Geometry check sheet. Reference: drawing and pictorial views, mm from the part's lowest x, y, z. A direction names the side the tool comes from. Round coordinates to 2 decimals unless told otherwise and drop trailing zeros. Write each loop counter-clockwise with the first axis right and the second up, starting at its lowest first coordinate (ties: lowest second). Pieces come first, ordered by that corner, then holes.
Item 1: Material ranges on line 1 along Y through (x, z) = (2.75, 3.25); line 2 along Z through (x, y) = (5.75, 1) (1 decimal); line 3 along X through (y, z) = (1.5, 6), recorded low to high.
Item 2: Section check D-D, the plane z = 4.25. Record the cut outline in (x, y).
Item 3: Section check C-C, the plane z = 6. Record the cut outline in (x, y).
Item 4: Release check for a two-part mould opening along Z. For the marked faces 3, 4, 5 and 6 record: pulls with the +Z half, pulls with the -Z half, needs draft (parallel to the pull), parting line crosses it, or undercut.
Item 5: Set-up check for the marked faces 1 and 2: record each of +Z, -Z, +X, -X, +Y, -Y from which the full face is reachable in a straight line by a thin tool's end or side.
Item 6: Depth check by flat-ended pin: pin 1 (3 mm diameter, centred on x = 6, y = 6.5, fed in from -Z). Enter the tip coordinate at first touch or a pass-through.
Item 7: Section check A-A, the plane x = 6.35. Record the cut outline in (y, z) (1 decimal).
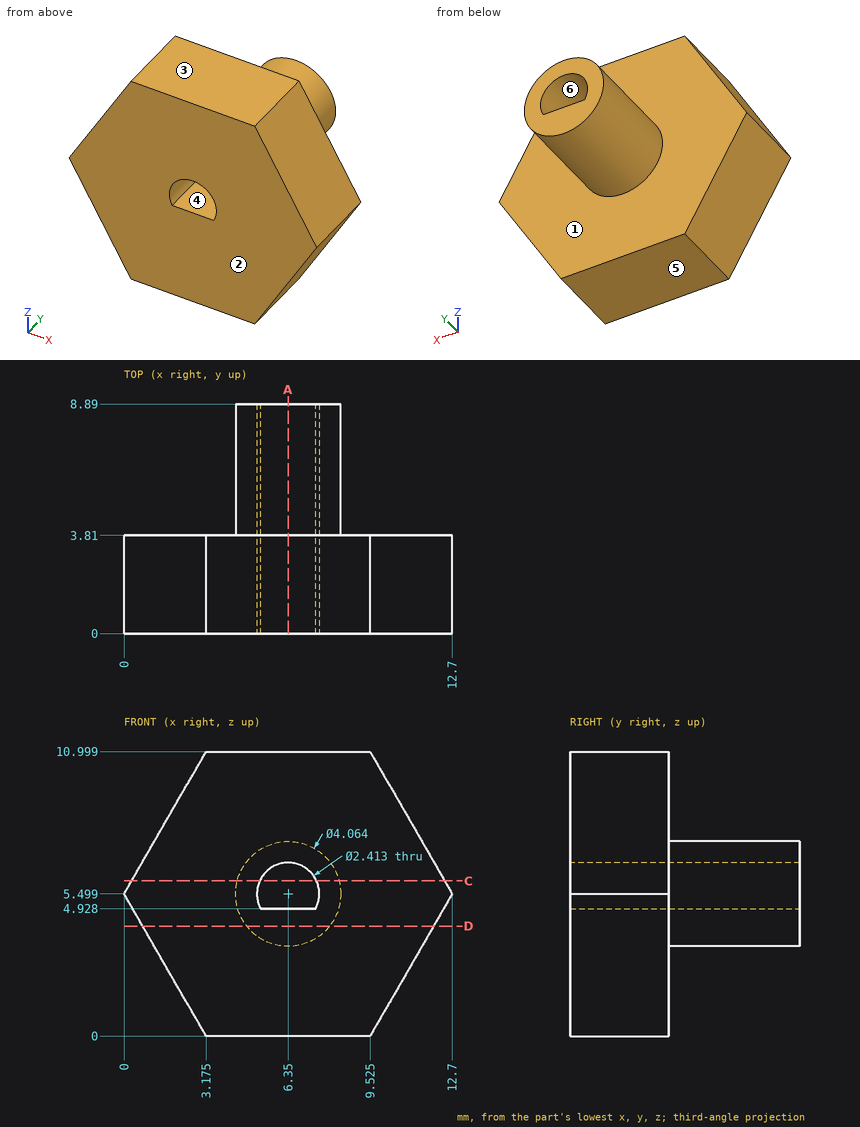
Values found:
1. line 1: y = 0 to 3.81
1. line 2: z = 0 to 4.9, 6.5 to 11
1. line 3: x = 0.29 to 5.25, 7.45 to 12.41
2. outline: (0.72, 0) - (11.98, 0) - (11.98, 3.81) - (7.95, 3.81) - (7.95, 8.89) - (4.75, 8.89) - (4.75, 3.81) - (0.72, 3.81) - close
3. outline: (0.29, 0) - (5.25, 0) - (5.25, 8.89) - (4.38, 8.89) - (4.38, 3.81) - (0.29, 3.81) - close; (7.45, 0) - (12.41, 0) - (12.41, 3.81) - (8.32, 3.81) - (8.32, 8.89) - (7.45, 8.89) - close
4. face 3: pulls with the +Z half
4. face 4: undercut
4. face 5: pulls with the -Z half
4. face 6: undercut
5. face 1: +Y
5. face 2: +Z, -Z, +X, -X, -Y
6. pin 1: stops at z = 3.47
7. outline: (0, 0) - (3.8, 0) - (3.8, 3.5) - (8.9, 3.5) - (8.9, 4.9) - (0, 4.9) - close; (0, 6.7) - (8.9, 6.7) - (8.9, 7.5) - (3.8, 7.5) - (3.8, 11) - (0, 11) - close
